Can you work these out from the model? Positions are in its coordinate system, mm. A direction names the side the tool comes from. Give positions to 0.01 mm unless a question says otherwise; leave off trailing zeros. Order: outer loops, then holes, each group sorted by start corner. A loop starts at its lowest first (then second) coordinate and runs counter-clockwise, first axis right, second up. Notation, with made-up numbers: (4.5, 68) -> (23.5, 68) arc R21 cw to (23.5, 106) -> close; hole circle Ø7 at (75.5, 23). An arc over 180 degrees is marked (long way). Answer as a JSON object with one key per item and string values.
Autodesk Fusion 360 part; units mm, degrees
sketch "Sketch1" plane through (0, 0, 0) normal (0, 0, 1) x (1, 0, 0)
  line L0 (18.5, 15) -> (-18.5, 15)
  line L1 (-18.5, 15) -> (-18.5, -15)
  line L2 (-18.5, -15) -> (18.5, -15)
  line L3 (18.5, -15) -> (18.5, 15)
  line L4 (18.5, 15) -> (-18.5, -15) construction
  line L5 (-18.5, 15) -> (18.5, -15) construction
  circle A0 centre (0, 0) radius 8
  circle A1 centre (0, 0) radius 5
  line L6 (-18.5, 15) -> (-15.5, 15)
  line L7 (-15.5, 15) -> (-15.5, -15)
  line L8 (-15.5, -15) -> (-18.5, -15)
  line L9 (-18.5, -15) -> (-18.5, 15)
  line L10 (-18.5, 15) -> (-15.5, -15) construction
  line L11 (-15.5, 15) -> (-18.5, -15) construction
  line L12 (0, 15) -> (0, -15) construction
  point P0 (-17, 0)
  dimension "d1" = 37
  dimension "d2" = 30
  dimension "d3" = 16
  dimension "d4" = 10
  dimension "d5" = 30
  dimension "d6" = 3
extrude "Extrude1" add sketch "Sketch1" against normal blind 10 contours L0 L1 L2 L6 L7 L8 L9 makes body 1
extrude "Extrude2" add sketch "Sketch1" along normal blind 3 separate body contours L0 L2 L3 L7 makes body 2
move_body "Move1" bodies 1 to x (1, 0, 0) y (0, 1, 0) z (0, 0, 1) at (3, 0, 0)
extrude "Extrude3" add sketch "Sketch1" along normal blind 23 contours A0 bodies 2
sketch "Sketch2" plane through (0, 0, 0) normal (1, 0, 0) x (0, 1, 0)
  line L0 (15, -5) -> (-15, -5) construction
  line L1 (15, -10) -> (-15, -10) construction
  line L2 (11, 3) -> (11, -10) construction
  line L3 (15, 3) -> (15, -10) construction
  line L4 (0, 3) -> (0, -10) construction
  circle A0 centre (11, -5) radius 1.6
  circle A1 centre (-11, -5) radius 1.6
  dimension "d13" = 5
  dimension "d14" = 13
  dimension "d15" = 4
  dimension "d16" = 3.2
extrude "Extrude4" cut sketch "Sketch2" against normal blind 20 contours A1 bodies 1
extrude "Extrude5" cut sketch "Sketch2" against normal blind 35 contours A0 bodies 1
sketch "Sketch3" plane through (0, 0, 0) normal (0, 1, 0) x (1, 0, 0)
  line L0 (-15.5, -3) -> (18.5, -3)
  dimension "d21" = 34
move_body "Move2" bodies 1 to x (1, 0, 0) y (0, 1, 0) z (0, 0, 1) at (-3, 0, 0)
extrude "Extrude6" add 1 faces at (-15.5, 5, 1) along direction (-1, 0, 0) blind 3 on bodies 2 bodies 1 2
sketch "Sketch4" plane through (0, 0, 0) normal (0, 1, 0) x (1, 0, 0)
sketch "Sketch5" plane through (0, 0, 0) normal (0, 0, 1) x (1, 0, 0)
  line L0 (-16, 0) -> (-19, 0) construction
1. For faces 4 (the face through (4.4, 6.9, 3)), 5 (the face through (-4, 15, 0.3)), 6 (the face through (-15.5, 0, -5)), which set-ups out of +Z, -Z, +X, -X, +Y, -Y let a thin tool reach every point of the face, with its end or its side?
Worked answers:
{"face 4": "+Z", "face 5": "+Z, -Z, +X, -X, +Y", "face 6": "-Z, +X, +Y, -Y"}
2. Will these pins go through, and if not, where does the flat tip stop? pin 1 Ø12 at (x, y) = (-5, -11.5) entering from -Z; pin 2 Ø1.9 at (y, z) = (11, -5) entering from +X; pin 3 Ø5 at (y, z) = (5, 13) entering from -X; pin 4 Ø4 at (y, z) = (3, 15) entering from -X.
Worked answers:
{"pin 1": "z = 0", "pin 2": "through", "pin 3": "x = -7.6", "pin 4": "x = -7.94"}
3. If we section it at D-D on y = 0: Please give me the cut outline in (x, z), then the cut area to 3 significant figures.
Worked answers:
{"outline": "(-18.5, -10) -> (-15.5, -10) -> (-15.5, 0) -> (-5, 0) -> (-5, 23) -> (-8, 23) -> (-8, 3) -> (-18.5, 3) -> close; (5, 0) -> (18.5, 0) -> (18.5, 3) -> (8, 3) -> (8, 23) -> (5, 23) -> close", "area": "231 mm²"}
4. If we mould it in two halves opening along Z, with no side actions, what happens to faces 1 (the face through (-16.98, -12.6, -4.93)), 2 (the face through (5, 4, 0)), 3 (the face through (-0.1, -5.2, 23))? For each: +Z half, -Z half, draft (parallel to the pull), parting line (faces both ways), or undercut.
Worked answers:
{"face 1": "undercut", "face 2": "-Z half", "face 3": "+Z half"}
5. If we section it at A-A on x = 0: Please give me the cut outline in (y, z), then the cut area to 3 significant figures.
Worked answers:
{"outline": "(-15, 0) -> (-5, 0) -> (-5, 23) -> (-8, 23) -> (-8, 3) -> (-15, 3) -> close; (5, 0) -> (15, 0) -> (15, 3) -> (8, 3) -> (8, 23) -> (5, 23) -> close", "area": "180 mm²"}
6. If we section it at C-C on z = -5: Please give me the cut outline in (x, y), then the cut area to 3 significant figures.
Worked answers:
{"outline": "(-18.5, -15) -> (-15.5, -15) -> (-15.5, -12.6) -> (-18.5, -12.6) -> close; (-18.5, -9.4) -> (-15.5, -9.4) -> (-15.5, 9.4) -> (-18.5, 9.4) -> close; (-18.5, 12.6) -> (-15.5, 12.6) -> (-15.5, 15) -> (-18.5, 15) -> close", "area": "70.8 mm²"}
7. Please list where these lines run through material, in increasing order: L1, parallel to Z at x = -17.35, y = -11; L2, parallel to Z at x = 3, y = -10.25; L3, parallel to X at y = 8.5, z = -6.
Worked answers:
{"L1": "-10 to -6.6, -3.4 to 3", "L2": "0 to 3", "L3": "-18.5 to -15.5"}
8. If we section it at B-B on y = 11: Please give me the cut outline in (x, z), then the cut area to 3 significant figures.
Worked answers:
{"outline": "(-18.5, -10) -> (-15.5, -10) -> (-15.5, -6.6) -> (-18.5, -6.6) -> close; (-18.5, -3.4) -> (-15.5, -3.4) -> (-15.5, 0) -> (18.5, 0) -> (18.5, 3) -> (-18.5, 3) -> close", "area": "131 mm²"}
